```python
from build123d import *

# Parameters (mm, degrees)
SKETCH1_W           = 120
SKETCH1_H           = 80
BOSS_EXTRUDE1_DEPTH = 10
SKETCH2_W           = 98
SKETCH2_H           = 40
CUT_EXTRUDE2_DEPTH  = 15
SKETCH4_R           = 1.5
CUT_EXTRUDE3_DEPTH  = 15
SKETCH5_W           = 120
SKETCH5_H           = 80
BOSS_EXTRUDE2_DEPTH = 5
SKETCH6_W           = 100
SKETCH6_H           = 60
CUT_EXTRUDE5_DEPTH  = 5


with BuildPart() as part:
    # Sketch1 → Boss-Extrude1 (new body)
    with BuildSketch(Plane.XY):
        Rectangle(SKETCH1_W, SKETCH1_H)
    extrude(amount=-BOSS_EXTRUDE1_DEPTH)

    # Sketch2 → Cut-Extrude2 (cut)
    with BuildSketch(Plane(origin=(0, 0, -10), x_dir=(-1, 0, 0), z_dir=(0, 0, -1))):
        Rectangle(SKETCH2_W, SKETCH2_H)
    extrude(amount=-CUT_EXTRUDE2_DEPTH, mode=Mode.SUBTRACT)

    # Sketch4 → Cut-Extrude3 (cut)
    with BuildSketch(Plane.XY):
        with Locations((-46.5, 27.5)):
            Circle(SKETCH4_R)
        with Locations((46.5, 27.5)):
            Circle(SKETCH4_R)
        with Locations((46.5, -27.5)):
            Circle(SKETCH4_R)
        with Locations((-46.5, -27.5)):
            Circle(SKETCH4_R)
    extrude(amount=-CUT_EXTRUDE3_DEPTH, mode=Mode.SUBTRACT)

    # Sketch5 → Boss-Extrude2 (add)
    with BuildSketch(Plane(origin=(0, 0, -10), x_dir=(-1, 0, 0), z_dir=(0, 0, -1))):
        Rectangle(SKETCH5_W, SKETCH5_H)
    extrude(amount=BOSS_EXTRUDE2_DEPTH)

    # Sketch6 → Cut-Extrude5 (cut)
    with BuildSketch(Plane(origin=(0, 0, -15), x_dir=(-1, 0, 0), z_dir=(0, 0, -1))):
        Rectangle(SKETCH6_W, SKETCH6_H)
    extrude(amount=-CUT_EXTRUDE5_DEPTH, mode=Mode.SUBTRACT)


solid = part.part
```
For this review, take the finished solid that the model builds, in its own axes (mm). A direction names the side the tool comes from. Round coordinates to 2 decimals unless told otherwise and drop trailing zeros. Write each loop counter-clockwise with the first axis right and the second up, starting at its lowest first coordinate (ties: lowest second). Pieces come first, ordered by that corner, then holes. Notation, with made-up numbers: (-2, 21) - (57, 21) arc R26 ccw to (57, 52) - close; hole circle Ø8 at (24.25, 84). An arc over 180 degrees is marked (long way). Answer as a JSON object with one key per item and string values.
1. We need section B-B on x = -46.5. Give the boundary of the cut face in (y, z).
Response values:
{"outline": "(-40, -15) - (-30, -15) - (-30, -10) - (-29, -10) - (-29, 0) - (-40, 0) - close; (-26, -10) - (-20, -10) - (-20, 0) - (-26, 0) - close; (20, -10) - (26, -10) - (26, 0) - (20, 0) - close; (29, -10) - (30, -10) - (30, -15) - (40, -15) - (40, 0) - (29, 0) - close"}
2. For pin 1 Ø4 at (x, y) = (-46.5, 27.5) entering from -Z; pin 2 Ø1.5 at (x, y) = (24, 18) entering from +Z, all flat-tipped, find the tip position at first contact; note any pin that passes through.
Response values:
{"pin 1": "stops at z = -10", "pin 2": "passes through"}
3. Draft analysis for pull direction Y (two halves, no side actions). For faces 1 (the face through (-49, 0, -5)), 2 (the face through (1, -40, -7)), 3 (the face through (-60, -1, -7)), state which applies: +Y half, -Y half, draft (parallel to the pull), parting line (faces both ways), or undercut.
Response values:
{"face 1": "undercut", "face 2": "-Y half", "face 3": "draft"}
4. To check wall thickness, follow line 1 along Y through (x, z) = (-46.5, -5); line 2 along Y through (x, z) = (5, -8.75); line 3 along X through (y, z) = (-18.5, -11.5). State the ranges of each line that lie inside material, in increasing order.
Response values:
{"line 1": "y = -40 to -29, -26 to -20, 20 to 26, 29 to 40", "line 2": "y = -40 to -20, 20 to 40", "line 3": "x = -60 to -50, 50 to 60"}
5. We need section C-C on z = -8. Give the boundary of the cut face in (x, y).
Response values:
{"outline": "(-60, -40) - (60, -40) - (60, 40) - (-60, 40) - close; hole (-49, -20) - (49, -20) - (49, 20) - (-49, 20) - close; hole circle Ø3 at (-46.5, -27.5); hole circle Ø3 at (-46.5, 27.5); hole circle Ø3 at (46.5, -27.5); hole circle Ø3 at (46.5, 27.5)"}
6. We need section D-D on x = 41. Give the boundary of the cut face in (y, z).
Response values:
{"outline": "(-40, -15) - (-30, -15) - (-30, -10) - (-20, -10) - (-20, 0) - (-40, 0) - close; (20, -10) - (30, -10) - (30, -15) - (40, -15) - (40, 0) - (20, 0) - close"}
7. We need section A-A on y = -27.5. Give the boundary of the cut face in (x, z), then the cut area to 3 significant figures.
Response values:
{"outline": "(-60, -15) - (-50, -15) - (-50, -10) - (-48, -10) - (-48, 0) - (-60, 0) - close; (-45, -10) - (45, -10) - (45, 0) - (-45, 0) - close; (48, -10) - (50, -10) - (50, -15) - (60, -15) - (60, 0) - (48, 0) - close", "area": "1,240 mm2"}
8. Tool access review of faces 4 (the face through (49, 0, -5)), 5 (the face through (0, 22, -10)), 6 (the face through (1, -35, -15)): name each direction out of +Z, -Z, +X, -X, +Y, -Y from which nothing blocks a thin tool from reaching the whole face with its end or side.
Response values:
{"face 4": "+Z, -Z", "face 5": "-Z", "face 6": "-Z, +X, -X, +Y, -Y"}
